from build123d import *

# Parameters (mm, degrees)
F1_DEPTH = 1.5
F3_DEPTH = 3
F5_DEPTH = 1.5
F6_W     = 4
F6_H     = 2.5
F7_DEPTH = 2.2


# Not quite as in the source:
# - a feature names something its author has since deleted; it is built from what else it names


with BuildPart() as f1:
    # F0 (on Top) → F1 (new body)
    with BuildSketch(Plane.XY):
        Polygon((10, 12), (-10, 12), (-10, -8), (-6, -8), (-6, 0), (6, 0), (6, -8), (10, -8), align=None)
    extrude(amount=F1_DEPTH)

    # F2 (on face) → F3 (join)
    with BuildSketch(Plane.XY.offset(1.5)):
        Polygon((-8, 5), (-8, -8), (-6, -8), (-6, 0), (6, 0), (6, -8), (8, -8), (8, 5), align=None)
    extrude(amount=F3_DEPTH)

    # F4 (on face) → F5 (join)
    with BuildSketch(Plane.XY.offset(4.5)):
        Polygon((-8, -8), (-6, -8), (-6, 0), (6, 0), (6, -8), (8, -8), (8, 5), (-8, 5), align=None)
        Polygon((-10, -8), (-8, -8), (-8, 5), (8, 5), (8, -8), (10, -8), (10, 12), (-10, 12), align=None)
    extrude(amount=F5_DEPTH)

    # F6 (on face) → F7 (cut)
    with BuildSketch(Plane.XY.offset(6)):
        with Locations((-8, -6.75)):
            Rectangle(F6_W, F6_H)
        with Locations((8, -6.75)):
            Rectangle(F6_W, F6_H)
    extrude(amount=-F7_DEPTH, mode=Mode.SUBTRACT)


solid = f1.part
Could you check a few things on this model? Use its own coordinates, in mm. A direction names the side the tool comes from. Give positions to 0.01 mm unless a question says otherwise; leave off trailing zeros. Order: outer loops, then holes, each group sorted by start corner. A loop starts at its lowest first (then second) coordinate and runs counter-clockwise, first axis right, second up. Notation, with made-up numbers: (76.5, 73.25) -> (97.5, 73.25) arc R34 ccw to (97.5, 112.25) -> close; hole circle Ø3 at (47, 78). An arc over 180 degrees is marked (long way). Answer in a Markdown table with one row per item. Add a question column.
Item 1: Imagine slicing it at B-B (z = 1.1). List the corners of the cut face in (x, y) for me.
Item 2: I'm going to push flat-ended pins straight in: P1, Ø1.1, axis at x = 8.5, z = 5, coming from the -Y side; P2, Ø2, axis at x = -7, y = -7, coming from the +Z side; P3, Ø1, axis at x = 4.5, y = -5, coming from the +Z side; P4, Ø1.5, axis at x = 0.5, z = 3, coming from the +Y side. Where does each tip first touch, or does it pass through?
Item 3: Please list where these lines run through material, in increasing order: probe 1 along Z at (x, y) = (-8.25, 8.5); probe 2 along X at (y, z) = (-3.5, 2.25); probe 3 along Y at (x, z) = (7, 5.75).
Item 4: We'd pull the mould along Z, two halves only. Please class faces 6 (the flat face through (0, 7, 4.5)), 7 (the flat face through (-6, -4, 3)), 8 (the flat face through (0, 5, 6)), 9 (the flat face through (8, -2, 3)): pulls with the +Z half, pulls with the -Z half, needs draft (parallel to the pull), parting line crosses it, or undercut.
Item 5: For faces 1 (the flat face through (-8, -1, 3)), 2 (the flat face through (6, -4, 3)), 3 (the flat face through (-8, -5.5, 5)), 4 (the flat face through (0, 12, 1)), 5 (the flat face through (0, 5, 3)), which set-ups out of +Z, -Z, +X, -X, +Y, -Y let a thin tool reach every point of the face, with its end or its side?
Item 6: Imagine slicing it at D-D (y = 4). List the corners of the cut face in (x, z) for me, and give its area (3 significant figures).
Item 7: Imagine slicing it at A-A (y = 8). List the corners of the cut face in (x, z) for me, and give its area (3 significant figures).
Item 8: Imagine slicing it at C-C (x = -7.5). List the corners of the cut face in (y, z) for me.
Result:
| question | item | result |
|---|---|---|
| 1 | outline | (-10, -8) -> (-6, -8) -> (-6, 0) -> (6, 0) -> (6, -8) -> (10, -8) -> (10, 12) -> (-10, 12) -> close |
| 2 | P1 | y = -5.5 |
| 2 | P2 | z = 3.8 |
| 2 | P3 | through |
| 2 | P4 | y = 5 |
| 3 | probe 1 | 0 to 1.5, 4.5 to 6 |
| 3 | probe 2 | -8 to -6, 6 to 8 |
| 3 | probe 3 | -5.5 to 12 |
| 4 | face 6 | undercut |
| 4 | face 7 | needs draft |
| 4 | face 8 | pulls with the +Z half |
| 4 | face 9 | undercut |
| 5 | face 1 | -X, +Y, -Y |
| 5 | face 2 | +Z, -Z, -Y |
| 5 | face 3 | +Z, +X, -X, -Y |
| 5 | face 4 | +Z, -Z, +X, -X, +Y |
| 5 | face 5 | +X, -X, +Y |
| 6 | outline | (-10, 0) -> (10, 0) -> (10, 1.5) -> (8, 1.5) -> (8, 4.5) -> (10, 4.5) -> (10, 6) -> (-10, 6) -> (-10, 4.5) -> (-8, 4.5) -> (-8, 1.5) -> (-10, 1.5) -> close |
| 6 | area | 108 mm2 |
| 7 | outline | (-10, 0) -> (10, 0) -> (10, 1.5) -> (-10, 1.5) -> close; (-10, 4.5) -> (10, 4.5) -> (10, 6) -> (-10, 6) -> close |
| 7 | area | 60.0 mm2 |
| 8 | outline | (-8, 0) -> (12, 0) -> (12, 1.5) -> (5, 1.5) -> (5, 4.5) -> (12, 4.5) -> (12, 6) -> (-5.5, 6) -> (-5.5, 3.8) -> (-8, 3.8) -> close |
